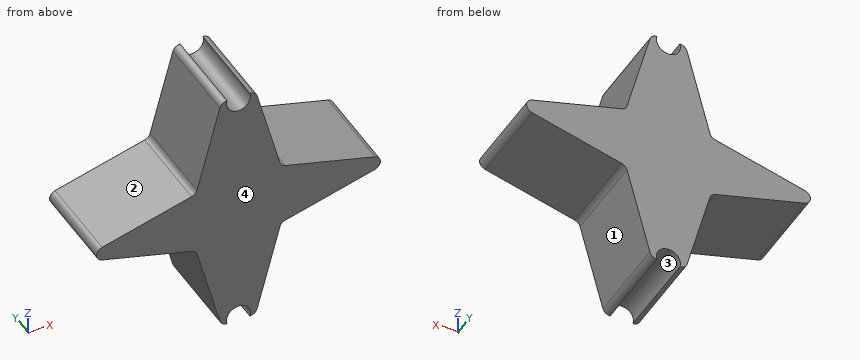
```python
from build123d import *

# Parameters (mm, degrees)
BOSS_EXTRU_1_DEPTH = 12


with BuildPart() as part:
    # Esquisse1 → Boss.-Extru.1 (new body)
    with BuildSketch(Plane(origin=(0, 0, 0), x_dir=(1, 0, 0), z_dir=(0, 1, 0))):
        with BuildLine():
            Line((2.485794242, 16.322649508), (5.549421558, 4.88903671))
            ThreePointArc((5.549421558, 4.88903671), (5.808240603, 4.440748973), (6.256528339, 4.181929928))
            Line((6.256528339, 4.181929928), (18.258819045, 0.965925826))
            ThreePointArc((18.258819045, 0.965925826), (19, 0), (18.258819045, -0.965925826))
            Line((18.258819045, -0.965925826), (6.256528339, -4.181929928))
            ThreePointArc((6.256528339, -4.181929928), (5.808240603, -4.440748973), (5.549421558, -4.88903671))
            Line((5.549421558, -4.88903671), (2.485794242, -16.322649508))
            ThreePointArc((2.485794242, -16.322649508), (2.128629844, -16.857183803), (1.519868415, -17.063830463))
            ThreePointArc((1.519868415, -17.063830463), (0, -14.963830463), (-1.519868415, -17.063830463))
            ThreePointArc((-1.519868415, -17.063830463), (-2.128629844, -16.857183803), (-2.485794242, -16.322649508))
            Line((-2.485794242, -16.322649508), (-5.549421558, -4.88903671))
            ThreePointArc((-5.549421558, -4.88903671), (-5.808240603, -4.440748973), (-6.256528339, -4.181929928))
            Line((-6.256528339, -4.181929928), (-18.258819045, -0.965925826))
            ThreePointArc((-18.258819045, -0.965925826), (-19, 0), (-18.258819045, 0.965925826))
            Line((-18.258819045, 0.965925826), (-6.256528339, 4.181929928))
            ThreePointArc((-6.256528339, 4.181929928), (-5.808240603, 4.440748973), (-5.549421558, 4.88903671))
            Line((-5.549421558, 4.88903671), (-2.485794242, 16.322649508))
            ThreePointArc((-2.485794242, 16.322649508), (-2.128629844, 16.857183803), (-1.519868415, 17.063830463))
            ThreePointArc((-1.519868415, 17.063830463), (0, 14.963830463), (1.519868415, 17.063830463))
            ThreePointArc((1.519868415, 17.063830463), (2.128629844, 16.857183803), (2.485794242, 16.322649508))
        make_face()
    extrude(amount=BOSS_EXTRU_1_DEPTH)


solid = part.part
```
Check sheet for the modelled part. Datum: model origin and axes. Units: mm. Face numbers are marked on the shaded views. Round coordinates to 2 decimals unless told otherwise and drop trailing zeros. Order: outer loops, then holes, each group sorted by start corner. A loop starts at its lowest first (then second) coordinate and runs counter-clockwise, first axis right, second up. Notation, with made-up numbers: M 63.5,-31.75 L 81.5,-31.75 A18 cw 81.5,-2.75 Z; hole C 49,-9 d3. An arc over 180 degrees is marked long. Answer in a Markdown table with one row per item.
(1) Section check A-A on y = 9.5. Record the boundary of the cut face in (x, z), plus the area to 3 significant figures.
Findings:
| item | result |
|---|---|
| outline | M -18.26,-0.97 L -6.26,-4.18 A1 cw -5.55,-4.89 L -2.49,-16.32 A1 ccw -1.52,-17.06 A1.6 cw long 1.52,-17.06 A1 ccw 2.49,-16.32 L 5.55,-4.89 A1 cw 6.26,-4.18 L 18.26,-0.97 A1 ccw 18.26,0.97 L 6.26,4.18 A1 cw 5.55,4.89 L 2.49,16.32 A1 ccw 1.52,17.06 A1.6 cw long -1.52,17.06 A1 ccw -2.49,16.32 L -5.55,4.89 A1 cw -6.26,4.18 L -18.26,0.97 A1 ccw Z |
| area | 426 mm^2 |
(2) Gauge pin test, flat ends, axial feed: pin 1 (8 mm diameter, centred on x = -10, z = 11, fed in from -Y); pin 2 (3 mm diameter, centred on y = 4.5, z = -10.5, fed in from -X); pin 3 (1 mm diameter, centred on y = 6, z = 6, fed in from -X). Record the tip position at first contact, or that the pin passes through.
Findings:
| item | result |
|---|---|
| pin 1 | passes through |
| pin 2 | stops at x = -4.45 |
| pin 3 | stops at x = -5.39 |
(3) Draft check along X on the marked faces 1, 2, 3 and 4. Enter one of: +X half, -X half, draft (parallel to the pull), parting line (faces both ways), or undercut.
Findings:
| item | result |
|---|---|
| face 1 | +X half |
| face 2 | -X half |
| face 3 | undercut |
| face 4 | draft |
(4) Material ranges on line 1 along X through (y, z) = (10.5, 7.5); line 2 along X through (y, z) = (9.5, -13.5); line 3 along Z through (x, y) = (-15, 0.5), recorded low to high. Write a range as from..to.
Findings:
| item | result |
|---|---|
| line 1 | x = -4.85..4.85 |
| line 2 | x = -3.24..3.24 |
| line 3 | z = -1.84..1.84 |
(5) Section check B-B on x = 0. Record the boundary of the cut face in (y, z).
Findings:
| item | result |
|---|---|
| outline | M 0,-14.96 L 12,-14.96 L 12,14.96 L 0,14.96 Z |
(6) Section check C-C on z = 11. Record the boundary of the cut face in (x, y).
Findings:
| item | result |
|---|---|
| outline | M -3.91,0 L 3.91,0 L 3.91,12 L -3.91,12 Z |
